Work out the finished part from the listing and answer in its coordinate system (mm). A direction names the side the tool comes from. Coordinates: 2 decimals unless noted, no trailing zeros. Order: outer loops, then holes, each group sorted by start corner. A loop starts at its lowest first (then second) coordinate and runs counter-clockwise, first axis right, second up.
1. The part is cut by section B-B, the plane z = -47. Give the vertices of the cut face in (x, y).
2. Flat-ended cylindrical pins translate along their axes: pin 1 Ø7.5 at (x, z) = (0, -28) entering from +Y; pin 2 Ø5 at (x, z) = (3.5, -45.5) entering from -Y. Find the tip coordinate at first contact, or state that the pin passes through.
3. The part is cut by section C-C, the plane z = -30. Give the vertices of the cut face in (x, y), then the cut area to 3 significant figures.
4. The part is cut by section D-D, the plane y = -3.75. Give the vertices of the cut face in (x, z).
5. Find the intervals of material crossed by probe 1 along X at (y, z) = (-0.6, -47); probe 2 along Z at (x, y) = (1, 0.75); probe 3 along X at (y, z) = (0.3, -28), in increasing order.
6. Determine the mould class of faces 4 (the flat face through (0, -1, -47)), 5 (the cylindrical face through (3.33, 0.014, -45.383)), 6 (the cylindrical face through (-0.119, -0.67, -1.617)), 7 (the flat face through (0, -2, -28)) for opening direction Y: +Y half, -Y half, draft (parallel to the pull), parting line (faces both ways), or undercut.
7. The part is cut by section A-A, the plane x = 0. Give the vertices of the cut face in (y, z), then the cut area to 3 significant figures.
8. A tool of negligible diameter and unlimited length cuts with its end or side. For faces 1 (the cylindrical face through (0.12, -4.14, 2.1)), 2 (the flat face through (0.1, -1.4, -42)), 3 (the flat face through (-0.75, 2, -47)), from which of +Z, -Z, +X, -X, +Y, -Y can it reach the whole face along a straight path? Write none if from no direction.
```python
from build123d import *

# Parameters (mm, degrees)
SKETCH1_R           = 1.75
BOSS_EXTRUDE1_DEPTH = 8.5
FILLET1_R           = 3
SKETCH2_R           = 1.75
CUT_EXTRUDE1_DEPTH  = 54.293995909
SKETCH2_3_R         = 1.75
CUT_EXTRUDE2_DEPTH  = 2
SKETCH3_R           = 4.25
CUT_EXTRUDE3_DEPTH  = 5


with BuildPart() as part:
    # Sketch1 → Boss-Extrude1 (new, symmetric)
    with BuildSketch(Plane(origin=(0, 0, 0), x_dir=(0, 0, -1), z_dir=(1, 0, 0))):
        with BuildLine():
            ThreePointArc((0, 3), (-2.121320344, 2.121320344), (-3, 0))
            Line((-3, 0), (-3, -5))
            Line((-3, -5), (6.279790789, -5))
            Line((6.279790789, -5), (42, -1.874886635))
            Line((42, -1.874886635), (42, -1))
            Line((42, -1), (52, -1))
            Line((52, -1), (52, 3))
            Line((52, 3), (0, 3))
        make_face()
        Circle(SKETCH1_R, mode=Mode.SUBTRACT)
    extrude(amount=BOSS_EXTRUDE1_DEPTH, both=True)

    # Fillet1
    fillet1_edges = [part.edges().sort_by_distance(p)[0] for p in [
        (0, -5, 3),
    ]]
    fillet(fillet1_edges, radius=FILLET1_R)

    # Sketch2 → Cut-Extrude1 (cut, through all)
    with BuildSketch(Plane(origin=(0, 3, 0), x_dir=(1, 0, 0), z_dir=(0, 1, 0))):
        with Locations(Location((-4, 47, 0), (0, 0, 270))):
            Circle(SKETCH2_R)
        with Locations(Location((4, 47, 0), (0, 0, 270))):
            Circle(SKETCH2_R)
    extrude(amount=-CUT_EXTRUDE1_DEPTH, mode=Mode.SUBTRACT)

    # Sketch2_3 → Cut-Extrude2 (cut)
    # profile 1 of 2: a face of its own
    with BuildSketch(Plane(origin=(0, 3, 0), x_dir=(1, 0, 0), z_dir=(0, 1, 0))):
        Polygon((4, 50.75277675), (0.75, 48.876388375), (0.75, 45.123611625), (4, 43.24722325), (7.25, 45.123611625), (7.25, 48.876388375), align=None)
        with Locations(Location((4, 47, 0), (0, 0, 270))):
            Circle(SKETCH2_3_R, mode=Mode.SUBTRACT)
    # profile 2 of 2: a face of its own
    with BuildSketch(Plane(origin=(0, 3, 0), x_dir=(1, 0, 0), z_dir=(0, 1, 0))):
        Polygon((-4, 43.24722325), (-0.75, 45.123611625), (-0.75, 48.876388375), (-4, 50.75277675), (-7.25, 48.876388375), (-7.25, 45.123611625), align=None)
        with Locations(Location((-4, 47, 0), (0, 0, 270))):
            Circle(SKETCH2_3_R, mode=Mode.SUBTRACT)
    extrude(amount=-CUT_EXTRUDE2_DEPTH, mode=Mode.SUBTRACT)

    # Sketch3 → Cut-Extrude3 (cut)
    with BuildSketch(Plane(origin=(0, 3, 0), x_dir=(1, 0, 0), z_dir=(0, 1, 0))):
        with Locations(Location((0, 28, 0), (0, 0, 270))):
            Circle(SKETCH3_R)
    extrude(amount=-CUT_EXTRUDE3_DEPTH, mode=Mode.SUBTRACT)


solid = part.part
```
Geometry says:
1. outline: (-8.5, -1) - (-5.75, -1) - (-5.75, 1) - (-7.25, 1) - (-7.25, 3) - (-8.5, 3) - close; (-2.25, -1) - (2.25, -1) - (2.25, 1) - (0.75, 1) - (0.75, 3) - (-0.75, 3) - (-0.75, 1) - (-2.25, 1) - close; (5.75, -1) - (8.5, -1) - (8.5, 3) - (7.25, 3) - (7.25, 1) - (5.75, 1) - close
2. pin 1: stops at y = -2
2. pin 2: stops at y = -1
3. outline: (-8.5, -2.92) - (8.5, -2.92) - (8.5, 3) - (3.75, 3) - (3.75, -2) - (-3.75, -2) - (-3.75, 3) - (-8.5, 3) - close
3. area: 63.2 mm2
4. outline: (-8.5, -20.57) - (8.5, -20.57) - (8.5, 2.44) - (-8.5, 2.44) - close
5. probe 1: x = -8.5 to -5.75, -2.25 to 2.25, 5.75 to 8.5
5. probe 2: z = -52 to -32.13, -23.87 to -1.58, 1.58 to 2.9
5. probe 3: x = -8.5 to -4.25, 4.25 to 8.5
6. face 4: -Y half
6. face 5: draft
6. face 6: undercut
6. face 7: +Y half
7. outline: (-5, -6.28) - (-1.87, -42) - (-1, -42) - (-1, -52) - (3, -52) - (3, -32.25) - (-2, -32.25) - (-2, -23.75) - (3, -23.75) - (3, 0) arc R3 ccw to (0, 3) - (-2, 3) arc R3 ccw to (-5, 0) - close; hole circle Ø3.5 at (0, 0)
7. area: 288 mm2
8. face 1: +Z, +X, -X, -Y
8. face 2: -Z, +X, -X, -Y
8. face 3: +Y
